Part model, mm, in its own coordinate system. Face numbers are marked on the shaded views. A direction names the side the tool comes from. Coordinates: 2 decimals unless noted, no trailing zeros. Loops run counter-clockwise (first coordinate to the right, second up) from the corner with the lowest first, then second, coordinate; pieces in that order, holes last.
```python
from build123d import *

# Parameters (mm, degrees)
F0_W     = 41.529
F0_H     = 38.989
F1_DEPTH = 1.27
F2_W     = 41.529
F2_H     = 38.989
F2_W_2   = 36.449
F2_H_2   = 33.909
F3_DEPTH = 9.525
F4_R     = 5.08
F5_R     = 1.27


with BuildPart() as f1:
    # F0 (on Top) → F1 (new body)
    with BuildSketch(Plane.XY):
        with Locations((1.983731, 4.818643)):
            Rectangle(F0_W, F0_H)
    extrude(amount=F1_DEPTH)

    # F2 (on face) → F3 (join)
    with BuildSketch(Plane.XY.offset(1.27)):
        with Locations((1.983731, 4.818643)):
            Rectangle(F2_W, F2_H)
        with Locations((1.983731, 4.818643)):
            Rectangle(F2_W_2, F2_H_2, mode=Mode.SUBTRACT)
    extrude(amount=F3_DEPTH)

    # F4
    f4_edges = [f1.edges().sort_by_distance(p)[0] for p in [
        (-18.780769, 24.313143, 5.3975),
        (22.748231, 24.313143, 5.3975),
        (22.748231, -14.675857, 5.3975),
        (-18.780769, -14.675857, 5.3975),
    ]]
    fillet(f4_edges, radius=F4_R)

    # F5
    f5_edges = [f1.edges().sort_by_distance(p)[0] for p in [
        (-16.240769, 21.773143, 6.0325),
        (20.208231, 21.773143, 6.0325),
        (20.208231, -12.135857, 6.0325),
        (-16.240769, -12.135857, 6.0325),
    ]]
    fillet(f5_edges, radius=F5_R)


solid = f1.part
```
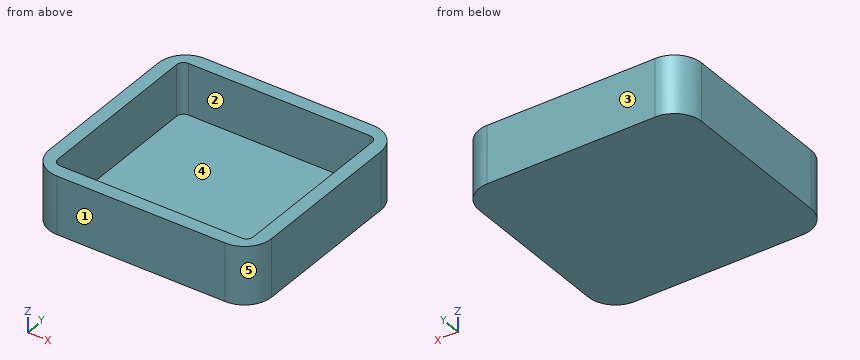
Q1. Saw through at A-A (x = 5). List the corners of the cut face in (y, z) (3 decimals).
Q2. Saw through at B-B (z = 5). List the corners of the cut face in (x, y).
Q3. Drop a flat-ended pin along its axis: P1, Ø10, axis at x = 7.5, y = 4.5, coming from the +Z side. Give the stop position or say it passes through.
Q4. Tool access for the marked faces 1 and 2: list every direction of +Z, -Z, +X, -X, +Y, -Y with a clear straight run to the whole face (end or side of a thin tool).
Q5. Mould opens along Y. For the marked faces 3, 4 and 5 say: released by +Y, released by -Y, zero draft, split by the parting line, or undercut.
Q6. Saw through at C-C (y = 12.5). List the corners of the cut face in (x, z) (3 decimals).
Q7. Probe line 1 (Y direction, x = -10, z = 2.5); line 2 (X direction, y = 19, z = 8.25); line 3 (Z direction, x = -10, y = -10). List the from-to ranges inside material, lowest first.
Checked values:
1. outline: (-14.676, 0) - (24.313, 0) - (24.313, 10.795) - (21.773, 10.795) - (21.773, 1.27) - (-12.136, 1.27) - (-12.136, 10.795) - (-14.676, 10.795) - close
2. outline: (-18.78, -9.6) arc R5.08 ccw to (-13.7, -14.68) - (17.67, -14.68) arc R5.08 ccw to (22.75, -9.6) - (22.75, 19.23) arc R5.08 ccw to (17.67, 24.31) - (-13.7, 24.31) arc R5.08 ccw to (-18.78, 19.23) - close; hole (-16.24, -10.87) arc R1.27 ccw to (-14.97, -12.14) - (18.94, -12.14) arc R1.27 ccw to (20.21, -10.87) - (20.21, 20.5) arc R1.27 ccw to (18.94, 21.77) - (-14.97, 21.77) arc R1.27 ccw to (-16.24, 20.5) - close
3. P1: stops at z = 1.27
4. face 1: +Z, -Z, +X, -X, -Y
4. face 2: +Z
5. face 3: released by +Y
5. face 4: undercut
5. face 5: released by -Y
6. outline: (-18.781, 0) - (22.748, 0) - (22.748, 10.795) - (20.208, 10.795) - (20.208, 1.27) - (-16.241, 1.27) - (-16.241, 10.795) - (-18.781, 10.795) - close
7. line 1: y = -14.68 to -12.14, 21.77 to 24.31
7. line 2: x = -18.78 to -16.24, 20.21 to 22.75
7. line 3: z = 0 to 1.27
